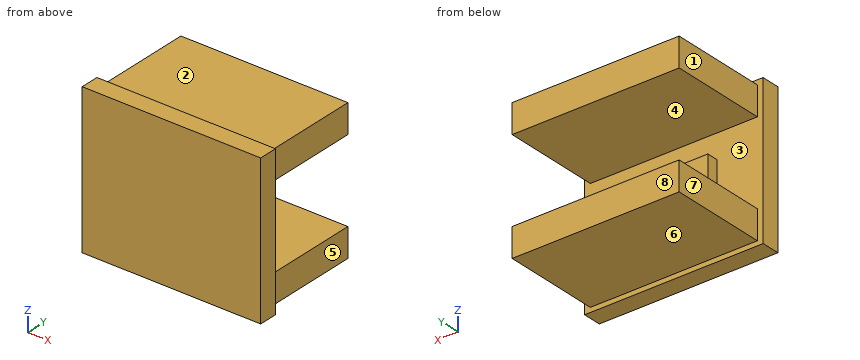
from build123d import *

# Parameters (mm, degrees)
SKETCH1_W       = 15.5
SKETCH1_H       = 13
PCB_DEPTH       = 1.6
HEADER_HV_START = 1.6
SKETCH2_W       = 14.5
SKETCH2_H       = 2.5
HEADER_HV_DEPTH = 8.5
HEADER_LV_START = 1.6
SKETCH3_W       = 14.5
SKETCH3_H       = 2.5
HEADER_LV_DEPTH = 8.5
MOSFETS_START   = 1.6
SKETCH4_W       = 7.5
SKETCH4_H       = 3
MOSFETS_DEPTH   = 1


with BuildPart() as part:
    # Sketch1 → PCB (new body)
    with BuildSketch(Plane(origin=(0, 0, 0), x_dir=(1, 0, 0), z_dir=(0, 1, 0))):
        with Locations((7.75, 6.5)):
            Rectangle(SKETCH1_W, SKETCH1_H)
    extrude(amount=PCB_DEPTH)

    # Sketch2 → Header_HV (add)
    with BuildSketch(Plane(origin=(0, 0, 0), x_dir=(1, 0, 0), z_dir=(0, 1, 0)).offset(HEADER_HV_START)):
        with Locations((7.75, 1.65)):
            Rectangle(SKETCH2_W, SKETCH2_H)
    extrude(amount=HEADER_HV_DEPTH)

    # Sketch3 → Header_LV (add)
    with BuildSketch(Plane(origin=(0, 0, 0), x_dir=(1, 0, 0), z_dir=(0, 1, 0)).offset(HEADER_LV_START)):
        with Locations((7.75, 11.35)):
            Rectangle(SKETCH3_W, SKETCH3_H)
    extrude(amount=HEADER_LV_DEPTH)

    # Sketch4 → MOSFETs (add)
    with BuildSketch(Plane(origin=(0, 0, 0), x_dir=(1, 0, 0), z_dir=(0, 1, 0)).offset(MOSFETS_START)):
        with Locations((7.75, 6.5)):
            Rectangle(SKETCH4_W, SKETCH4_H)
    extrude(amount=MOSFETS_DEPTH)


solid = part.part
Input: part model. Units: mm. Frame: model coordinates. Face numbers are marked on the shaded views. A direction names the side the tool comes from. Give positions to 0.01 mm unless a question says otherwise; leave off trailing zeros. Order: outer loops, then holes, each group sorted by start corner. A loop starts at its lowest first (then second) coordinate and runs counter-clockwise, first axis right, second up. Notation, with made-up numbers: M 33.5,59 L 66.5,59 A19 cw 66.5,90 Z; hole C -4,32 d8. An arc over 180 degrees is marked long. Answer as a JSON object with one key per item and string values.
1. First-contact query: P1, Ø4, axis at x = 10.5, y = 6.5, coming from the -Z side; P2, Ø6, axis at y = 8.5, z = -1.5, coming from the +X side; P3, Ø4, axis at x = 10, y = 7.5, coming from the +Z side. Flat tips, straight axial feed; report the tip coordinate or a pass-through.
Result sheet:
{"P1": "z = -12.6", "P2": "x = 15", "P3": "z = -0.4"}
2. Ray query, line 1 (Z direction, x = 8, y = 2.5); line 2 (Z direction, x = 13, y = 7.5); line 3 (X direction, y = 9, z = -12.5). Return the intervals inside material, ascending. Write a range as [from, to].
Result sheet:
{"line 1": "[-12.6, -10.1], [-8, -5], [-2.9, -0.4]", "line 2": "[-12.6, -10.1], [-2.9, -0.4]", "line 3": "[0.5, 15]"}
3. Cut plane A-A, the plane y = 3.25. Output: boundary loops of the cut face in (x, z), and give its area (3 significant figures).
Result sheet:
{"outline": "M 0.5,-12.6 L 15,-12.6 L 15,-10.1 L 0.5,-10.1 Z; M 0.5,-2.9 L 15,-2.9 L 15,-0.4 L 0.5,-0.4 Z", "area": "72.5 mm²"}
4. Reachability of the marked faces 4, 5, 6, 7 and 8 from +Z, -Z, +X, -X, +Y, -Y: full face, straight path, thin tool, end or side. Return the list, or none.
Result sheet:
{"face 4": "+X, -X, +Y", "face 5": "+Z, -Z, +X, +Y", "face 6": "-Z, +X, -X, +Y", "face 7": "+Z, -Z, -X, +Y", "face 8": "+Z, -Z, +X, -X, +Y"}
5. Cut plane B-B, the plane x = 12. Output: boundary loops of the cut face in (y, z).
Result sheet:
{"outline": "M 0,-13 L 1.6,-13 L 1.6,-12.6 L 10.1,-12.6 L 10.1,-10.1 L 1.6,-10.1 L 1.6,-2.9 L 10.1,-2.9 L 10.1,-0.4 L 1.6,-0.4 L 1.6,0 L 0,0 Z"}
6. Cut plane D-D, the plane x = 9.5. Output: boundary loops of the cut face in (y, z), and give its area (3 significant figures).
Result sheet:
{"outline": "M 0,-13 L 1.6,-13 L 1.6,-12.6 L 10.1,-12.6 L 10.1,-10.1 L 1.6,-10.1 L 1.6,-8 L 2.6,-8 L 2.6,-5 L 1.6,-5 L 1.6,-2.9 L 10.1,-2.9 L 10.1,-0.4 L 1.6,-0.4 L 1.6,0 L 0,0 Z", "area": "66.3 mm²"}
7. Pull-direction query (Z, two-part tool) for the marked faces 1, 2 and 3; classes: +Z half, -Z half, draft (parallel to the pull), parting line (faces both ways), or undercut.
Result sheet:
{"face 1": "draft", "face 2": "+Z half", "face 3": "undercut"}
8. Cut plane C-C, the plane z = -7. Output: boundary loops of the cut face in (x, y), and give its area (3 significant figures).
Result sheet:
{"outline": "M 0,0 L 15.5,0 L 15.5,1.6 L 11.5,1.6 L 11.5,2.6 L 4,2.6 L 4,1.6 L 0,1.6 Z", "area": "32.3 mm²"}
